from build123d import *

# Parameters (mm, degrees)
SKETCH2_R          = 3.5
SKETCH2_R_2        = 1.5
BASE_FLANGE1_DEPTH = 1
CHAMFER1_SIZE      = 0.25


# Sheet-metal steps are written as plain solids
with BuildPart() as part:
    # Sketch2 → Base-Flange1 (new body)
    with BuildSketch(Plane.XY):
        Circle(SKETCH2_R)
        Circle(SKETCH2_R_2, mode=Mode.SUBTRACT)
    extrude(amount=-BASE_FLANGE1_DEPTH)

    # Chamfer1
    chamfer1_edges = [part.edges().sort_by_distance(p)[0] for p in [
        (-3.5, 0, 0),
        (-3.5, 0, -1),
        (-1.5, 0, -1),
        (-1.5, 0, 0),
    ]]
    chamfer(chamfer1_edges, length=CHAMFER1_SIZE)


solid = part.part
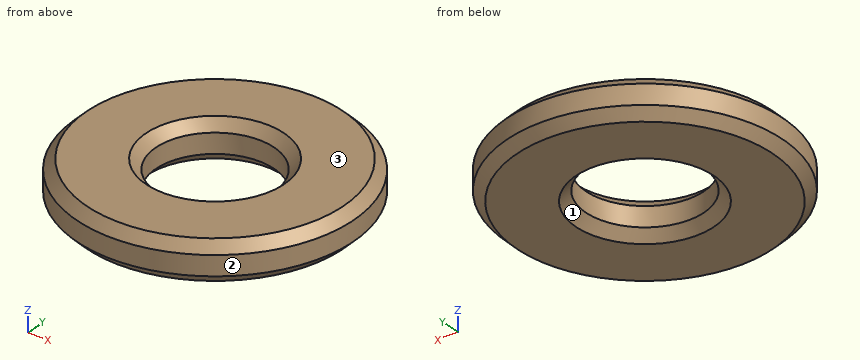
The listing builds one solid part. Answer for the finished solid, in the listing's coordinates (mm). Face numbers are marked on the shaded views. Round coordinates to 2 decimals unless told otherwise and drop trailing zeros. Loops run counter-clockwise (first coordinate to the right, second up) from the corner with the lowest first, then second, coordinate; pieces in that order, holes last. Notation, with made-up numbers: M 61.25,-14 L 70.25,-14 A34 cw 70.25,21 Z; hole C -14,47 d10. An arc over 180 degrees is marked long. Write each question's results on one line, items separated by ' | '. Start each with the question number.
1) Find section A-A on y = 0. Write down the section's boundary in (x, z), plus the area to 3 significant figures.
2) This flat-tipped pin is pushed along its axis until it touches: pin 1 (2.5 mm diameter, centred on x = 0, y = 0, fed in from +Z). Where does it stop, or does it pass through?
3) Straight lines are drawn through the part: probe 1 along Y at (x, z) = (0, -0.4); probe 2 along X at (y, z) = (-0.25, -0.7); probe 3 along Y at (x, z) = (0.25, -0.9). For each, find the intervals that lie inside material, in ascending order.
4) Find section C-C on z = -0.5. Write down the section's boundary in (x, y).
5) Determine the mould class of the marked faces 1, 2 and 3 for opening direction Y: pulls with the +Y half, pulls with the -Y half, needs draft (parallel to the pull), parting line crosses it, or undercut.
Final values:
1) outline: M -3.5,-0.75 L -3.25,-1 L -1.75,-1 L -1.5,-0.75 L -1.5,-0.25 L -1.75,0 L -3.25,0 L -3.5,-0.25 Z; M 1.5,-0.75 L 1.75,-1 L 3.25,-1 L 3.5,-0.75 L 3.5,-0.25 L 3.25,0 L 1.75,0 L 1.5,-0.25 Z | area: 3.75 mm²
2) pin 1: through
3) probe 1: -3.5 to -1.5, 1.5 to 3.5 | probe 2: -3.49 to -1.48, 1.48 to 3.49 | probe 3: -3.34 to -1.63, 1.63 to 3.34
4) outline: C 0,0 d7; hole C 0,0 d3
5) face 1: undercut | face 2: parting line crosses it | face 3: needs draft
